from build123d import *

# Parameters (mm, degrees)
SKETCH_1_W             = 45
SKETCH_1_H             = 20
SKETCH_1_R             = 0.75
EXTRUDE_1_DEPTH        = 1.3
SKETCH_2_R             = 8
EXTRUDE_2_DEPTH        = 12
SKETCH_3_W             = 2.5
SKETCH_3_H             = 2.5
EXTRUDE_3_DEPTH        = 2.5
SKETCH_5_W             = 0.6
SKETCH_5_H             = 0.6
PATTERN_LINEAR_3_COUNT = 4
PATTERN_LINEAR_3_PITCH = 2.54


with BuildPart() as part:
    # 草图1 → 凸台-拉伸1 (new body)
    with BuildSketch(Plane.XY):
        Rectangle(SKETCH_1_W, SKETCH_1_H)
        with Locations((-21.25, 8.75)):
            Circle(SKETCH_1_R, mode=Mode.SUBTRACT)
        with Locations((21.25, 8.75)):
            Circle(SKETCH_1_R, mode=Mode.SUBTRACT)
        with Locations((21.25, -8.75)):
            Circle(SKETCH_1_R, mode=Mode.SUBTRACT)
        with Locations((-21.25, -8.75)):
            Circle(SKETCH_1_R, mode=Mode.SUBTRACT)
    extrude(amount=EXTRUDE_1_DEPTH)

    # 草图2 → 凸台-拉伸2 (add)
    with BuildSketch(Plane.XY.offset(1.3)):
        with Locations((-13, 0)):
            Circle(SKETCH_2_R)
        with Locations((13, 0)):
            Circle(SKETCH_2_R)
    extrude(amount=EXTRUDE_2_DEPTH)

    # 草图3 → 凸台-拉伸3 (add)
    with BuildSketch(Plane(origin=(0, 0, 0), x_dir=(-1, 0, 0), z_dir=(0, 0, -1))):
        with Locations((3.75, -8.75)):
            Rectangle(SKETCH_3_W, SKETCH_3_H)
    extrude_3 = extrude(amount=EXTRUDE_3_DEPTH)

    # 扫描1: sweep along a path in 草图4
    with BuildLine(Plane.ZY.offset(3.75)) as sweep_1_path:
        Line((-2.5, -8.75), (-3.2, -8.75))
        ThreePointArc((-3.2, -8.75), (-3.553553391, -8.896446609), (-3.7, -9.25))
        Line((-3.7, -9.25), (-3.7, -16.45))
    # 草图5 → 扫描1 (sweep)
    with BuildSketch(Plane(origin=(0, 0, -2.5), x_dir=(-1, 0, 0), z_dir=(0, 0, -1))):
        with Locations((3.75, -8.75)):
            Rectangle(SKETCH_5_W, SKETCH_5_H)
    sweep_1 = sweep(path=sweep_1_path.line)

    # 阵列(线性)3: 凸台-拉伸3, 扫描1 ×4
    with Locations(*[(i * PATTERN_LINEAR_3_PITCH, 0, 0) for i in range(1, PATTERN_LINEAR_3_COUNT)]):
        add(extrude_3)
        add(sweep_1)


solid = part.part
Can you work these out from the model? Positions are in its coordinate system, mm. A direction names the side the tool comes from. Round coordinates to 2 decimals unless told otherwise and drop trailing zeros. Write each loop counter-clockwise with the first axis right and the second up, starting at its lowest first coordinate (ties: lowest second). Pieces come first, ordered by that corner, then holes. Notation, with made-up numbers: (47, 7) - (71, 7) arc R12 ccw to (71, 17) - close; hole circle Ø4 at (60.25, -3). An arc over 180 degrees is marked (long way). Write each question's results on one line, items separated by ' | '. Start each with the question number.
1) Suppose I cut it at C-C (x = 13). List the corners of the cut face in (y, z) for me, and give its area (3 significant figures).
2) For pin 1 Ø3 at (x, y) = (11, -9.5) entering from -Z; pin 2 Ø6 at (y, z) = (4, 10.5) entering from -X; pin 3 Ø1.2 at (x, y) = (2, -8.5) entering from -Z, each with a flat end and sliding along its axis, tell me the tip position at first contact or that it passes through.
3) Suppose I cut it at B-B (y = -12). List the corners of the cut face in (x, z) for me, and give its area (3 significant figures).
4) Suppose I cut it at D-D (y = 0). List the corners of the cut face in (x, z) for me, and give its area (4 significant figures).
5) Suppose I cut it at A-A (z = -1.25). List the corners of the cut face in (x, y) for me, and give its area (3 significant figures).
6) Please list where these lines run through material, in increasing order: line 1 (Y direction, x = -21.25, z = 0.6); line 2 (X direction, y = 8.25, z = 1.25); line 3 (Z direction, x = -19.5, y = 1).
7) Which directions (+Z, -Z, +X, -X, +Y, -Y) give clear straight access to the entire face, cutting with the end or side of a thin tool? Please do faces 5 (the flat face through (-1, -7.5, -1)), 6 (the cylindrical face through (-14.73, -7.81, 7.22)), 7 (the flat face through (-4, -8, -2.5)).
8) We'd pull the mould along X, two halves only. Please class faces 1 (the flat face through (-3.45, -12.4, -3.6)), 2 (the flat face through (-1.51, -12.5, -3.6)), 3 (the flat face through (-13, 0, 13.3)), 4 (the flat face through (-22.5, 0, 1)): released by +X, released by -X, zero draft, split by the parting line, or undercut.
Here are the results:
1) outline: (-10, 0) - (10, 0) - (10, 1.3) - (8, 1.3) - (8, 13.3) - (-8, 13.3) - (-8, 1.3) - (-10, 1.3) - close | area: 218 mm2
2) pin 1: stops at z = 0 | pin 2: stops at x = -20.94 | pin 3: stops at z = -3.95
3) outline: (-4.05, -4) - (-3.45, -4) - (-3.45, -3.4) - (-4.05, -3.4) - close; (-1.51, -4) - (-0.91, -4) - (-0.91, -3.4) - (-1.51, -3.4) - close; (1.03, -4) - (1.63, -4) - (1.63, -3.4) - (1.03, -3.4) - close; (3.57, -4) - (4.17, -4) - (4.17, -3.4) - (3.57, -3.4) - close | area: 1.44 mm2
4) outline: (-22.5, 0) - (22.5, 0) - (22.5, 1.3) - (21, 1.3) - (21, 13.3) - (5, 13.3) - (5, 1.3) - (-5, 1.3) - (-5, 13.3) - (-21, 13.3) - (-21, 1.3) - (-22.5, 1.3) - close | area: 442.5 mm2
5) outline: (-5, -10) - (-2.5, -10) - (-2.5, -7.5) - (-5, -7.5) - close; (-2.46, -10) - (0.04, -10) - (0.04, -7.5) - (-2.46, -7.5) - close; (0.08, -10) - (2.58, -10) - (2.58, -7.5) - (0.08, -7.5) - close; (2.62, -10) - (5.12, -10) - (5.12, -7.5) - (2.62, -7.5) - close | area: 25.0 mm2
6) line 1: y = -10 to -9.5, -8 to 8, 9.5 to 10 | line 2: x = -22.5 to -21.81, -20.69 to 20.69, 21.81 to 22.5 | line 3: z = 0 to 13.3
7) face 5: -Z, +X, -X, +Y | face 6: +Z | face 7: none
8) face 1: undercut | face 2: undercut | face 3: zero draft | face 4: released by -X
